```python
from build123d import *

# Parameters (mm, degrees)
SKETCH1_W           = 25.4
SKETCH1_H           = 25.4
BOSS_EXTRUDE1_DEPTH = 25.4
CUT_EXTRUDE1_START  = -2
SKETCH2_R           = 7.5
CUT_EXTRUDE1_DEPTH  = 42.994090512
CUT_EXTRUDE3_START  = -2
SKETCH4_R           = 7.5
CUT_EXTRUDE3_DEPTH  = 42.994090512
SKETCH5_R           = 3.75
CUT_EXTRUDE4_DEPTH  = 43.87050268
SKETCH7_R           = 3.75
CUT_EXTRUDE6_DEPTH  = 43.87050268
SKETCH6_R           = 3.75
CUT_EXTRUDE7_DEPTH  = 10
CUT_EXTRUDE8_START  = 2
SKETCH3_R           = 7.5
CUT_EXTRUDE8_DEPTH  = 42.994090628


with BuildPart() as part:
    # Sketch1 → Boss-Extrude1 (new body)
    with BuildSketch(Plane.XY):
        with Locations((12.7, 12.7)):
            Rectangle(SKETCH1_W, SKETCH1_H)
    extrude(amount=BOSS_EXTRUDE1_DEPTH)

    # Sketch2 → Cut-Extrude1 (cut, through all)
    with BuildSketch(Plane(origin=(0, 0, 0), x_dir=(-1, 0, 0), z_dir=(0, 0, -1)).offset(CUT_EXTRUDE1_START)):
        with Locations((-12.7, 12.7)):
            Circle(SKETCH2_R)
    extrude(amount=-CUT_EXTRUDE1_DEPTH, mode=Mode.SUBTRACT)

    # Sketch4 → Cut-Extrude3 (cut, through all)
    with BuildSketch(Plane.XZ.offset(CUT_EXTRUDE3_START)):
        with Locations(Location((12.7, 12.7, 0), (0, 0, 270))):
            Circle(SKETCH4_R)
    extrude(amount=-CUT_EXTRUDE3_DEPTH, mode=Mode.SUBTRACT)

    # Sketch5 → Cut-Extrude4 (cut, through all)
    with BuildSketch(Plane(origin=(0, 2, 0), x_dir=(1, 0, 0), z_dir=(0, 1, 0))):
        with Locations(Location((12.7, -12.7, 0), (0, 0, 270))):
            Circle(SKETCH5_R)
    extrude(amount=-CUT_EXTRUDE4_DEPTH, mode=Mode.SUBTRACT)

    # Sketch7 → Cut-Extrude6 (cut, through all)
    with BuildSketch(Plane.XY.offset(2)):
        with Locations((12.7, 12.7)):
            Circle(SKETCH7_R)
    extrude(amount=-CUT_EXTRUDE6_DEPTH, mode=Mode.SUBTRACT)

    # Sketch6 → Cut-Extrude7 (cut)
    with BuildSketch(Plane.ZY):
        with Locations((12.7, 12.7)):
            Circle(SKETCH6_R)
    extrude(amount=-CUT_EXTRUDE7_DEPTH, mode=Mode.SUBTRACT)

    # Sketch3 → Cut-Extrude8 (cut, through all)
    with BuildSketch(Plane(origin=(0, 0, 0), x_dir=(0, 0, -1), z_dir=(1, 0, 0)).offset(CUT_EXTRUDE8_START)):
        with Locations((-12.7, 12.7)):
            Circle(SKETCH3_R)
    extrude(amount=CUT_EXTRUDE8_DEPTH, mode=Mode.SUBTRACT)


solid = part.part
```
For this review, take the finished solid that the model builds, in its own axes (mm). A direction names the side the tool comes from. Coordinates: 2 decimals unless noted, no trailing zeros. Write each loop counter-clockwise with the first axis right and the second up, starting at its lowest first coordinate (ties: lowest second). Pieces come first, ordered by that corner, then holes. Notation, with made-up numbers: (-1.75, -25.5) -> (20.25, -25.5) arc R30 ccw to (20.25, -1.5) -> close; hole circle Ø9 at (52.25, 71). An arc over 180 degrees is marked (long way). Put each result on its own line as item: value.
Q1. Take a section at C-C, the plane x = 6.75. State the section outline as (y, z) points, then the cut area to 3 significant figures.
From the geometry:
outline: (0, 0) -> (25.4, 0) -> (25.4, 8.13) -> (18.65, 8.13) arc R7.5 cw to (17.27, 6.75) -> (17.27, 2) -> (8.13, 2) -> (8.13, 6.75) arc R7.5 cw to (6.75, 8.13) -> (2, 8.13) -> (2, 17.27) -> (6.75, 17.27) arc R7.5 cw to (8.13, 18.65) -> (8.13, 25.4) -> (0, 25.4) -> close; (17.27, 18.65) arc R7.5 cw to (18.65, 17.27) -> (25.4, 17.27) -> (25.4, 25.4) -> (17.27, 25.4) -> close
area: 297 mm2
Q2. Tool access review of faces 1 (the flat face through (9, 9, 2)), 2 (the flat face through (25.4, 18, 7)), 3 (the flat face through (9, 2, 9)), 4 (the flat face through (2, 9, 9)): name each direction out of +Z, -Z, +X, -X, +Y, -Y from which nothing blocks a thin tool from reaching the whole face with its end or side.
From the geometry:
face 1: +Z
face 2: +Z, -Z, +X, +Y, -Y
face 3: +Y
face 4: +X
Q3. Take a section at D-D, the plane y = 2.5. State the section outline as (x, z) points.
From the geometry:
outline: (0, 0) -> (25.4, 0) -> (25.4, 25.4) -> (0, 25.4) -> close; hole circle Ø15 at (12.7, 12.7)
Q4. Wall thickness on L1, parallel to X at y = 4.4, z = 12.7; L2, parallel to Y at x = 21, z = 13; L3, parallel to X at y = 6.5, z = 24.5: over which ranges is each line inside the solid? List them lowest first.
From the geometry:
L1: x = 0 to 5.2, 20.2 to 25.4
L2: y = 0 to 5.21, 20.19 to 25.4
L3: x = 0 to 8.48, 16.92 to 25.4
Q5. Clearance check with flat-ended pins moving along their axes: pin 1 Ø10 at (x, y) = (12.7, 12.7) entering from +Z; pin 2 Ø1.5 at (y, z) = (16, 18) entering from +X. State where each tip first meets the part, or that it passes through.
From the geometry:
pin 1: stops at z = 2
pin 2: stops at x = 2
Q6. The part is to be moulded in two halves that separate along Z. For faces 5 (the flat face through (10, 16, 0)), 6 (the cylindrical face through (13.03, 4.061, 20.193)), 7 (the cylindrical face through (20.136, 22.472, 13.676)), 8 (the cylindrical face through (14.43, 9.373, 1.014)), say which applies: +Z half, -Z half, draft (parallel to the pull), parting line (faces both ways), or undercut.
From the geometry:
face 5: -Z half
face 6: undercut
face 7: undercut
face 8: draft
Q7. Take a section at A-A, the plane z = 12.7. State the section outline as (x, y) points.
From the geometry:
outline: (0, 0) -> (8.95, 0) -> (8.95, 2) -> (5.2, 2) -> (5.2, 5.2) -> (2, 5.2) -> (2, 8.95) -> (0, 8.95) -> close; (0, 16.45) -> (2, 16.45) -> (2, 20.2) -> (5.2, 20.2) -> (5.2, 25.4) -> (0, 25.4) -> close; (16.45, 0) -> (25.4, 0) -> (25.4, 5.2) -> (20.2, 5.2) -> (20.2, 2) -> (16.45, 2) -> close; (20.2, 20.2) -> (25.4, 20.2) -> (25.4, 25.4) -> (20.2, 25.4) -> close
